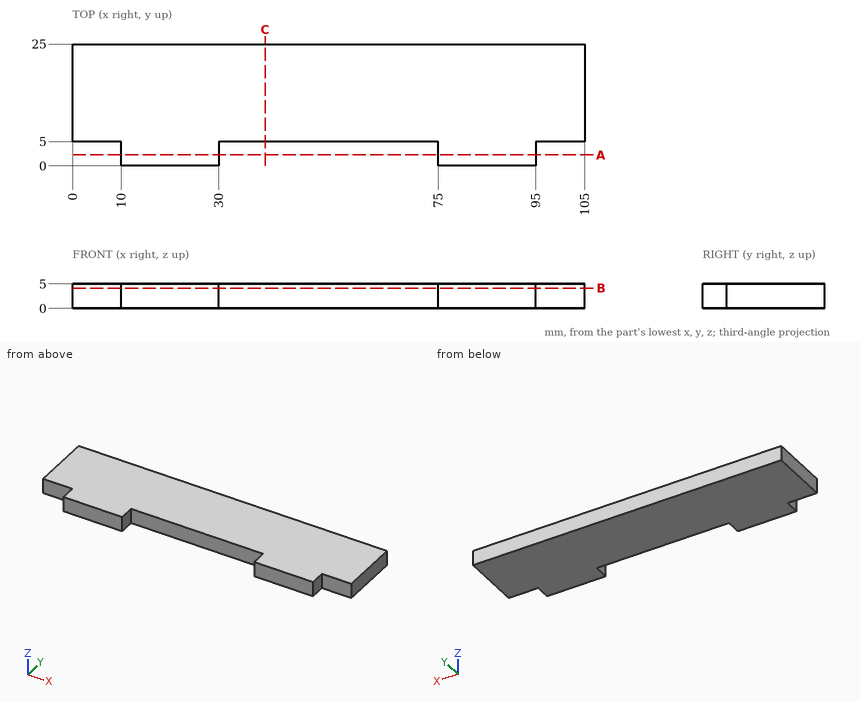
Source: three-view drawing plus pictorial views. Frame: mm from the lowest corner of the part. Give positions to 0.01 mm unless a question says otherwise; leave off trailing zeros. Loops run counter-clockwise (first coordinate to the right, second up) from the corner with the lowest first, then second, coordinate; pieces in that order, holes last.
1) Line query: L1, parallel to X at y = 4, z = 2.75; L2, parallel to Y at x = 74, z = 4.35. Output: solid intervals per line, ascending.
A:
L1: x = 10 to 30, 75 to 95
L2: y = 5 to 25
2) Contact query for flat-ended pins moving along their axis: pin 1 (1.5 mm diameter, centred on y = 2, z = 2.5, fed in from -X); pin 2 (1.5 mm diameter, centred on y = 2, z = 3.5, fed in from +X); pin 3 (1.5 mm diameter, centred on x = 53.5, z = 2.5, fed in from -Y). Output: stop coordinate, or through.
A:
pin 1: stops at x = 10
pin 2: stops at x = 95
pin 3: stops at y = 5
3) Section query B-B on z = 4.15. Return the cut outline in (x, y), and give its area (3 significant figures).
A:
outline: (0, 5) - (10, 5) - (10, 0) - (30, 0) - (30, 5) - (75, 5) - (75, 0) - (95, 0) - (95, 5) - (105, 5) - (105, 25) - (0, 25) - close
area: 2,300 mm2
4) Section query A-A on y = 2.25. Return the cut outline in (x, z), and give its area (3 significant figures).
A:
outline: (10, 0) - (30, 0) - (30, 5) - (10, 5) - close; (75, 0) - (95, 0) - (95, 5) - (75, 5) - close
area: 200 mm2
5) Section query C-C on x = 39.5. Return the cut outline in (y, z), and give its area (3 significant figures).
A:
outline: (5, 0) - (25, 0) - (25, 5) - (5, 5) - close
area: 100 mm2
